```python
from build123d import *

# Parameters (mm, degrees)
CYLINDER001_R     = 5
CYLINDER001_DEPTH = 1.5
CYLINDER002_R     = 2.2
CYLINDER002_DEPTH = 5
CYLINDER_R        = 3
CYLINDER_DEPTH    = 5


with BuildPart() as cylinder001:
    # Cylinder001 → Cylinder001 (new body)
    with BuildSketch(Plane.XY.offset(5)):
        Circle(CYLINDER001_R)
    extrude(amount=CYLINDER001_DEPTH)


with BuildPart() as cylinder002:
    # Cylinder002 → Cylinder002 (new body)
    with BuildSketch(Plane.XY):
        Circle(CYLINDER002_R)
    extrude(amount=CYLINDER002_DEPTH)


with BuildPart() as fusion001:
    # Cylinder → Cylinder (new body)
    with BuildSketch(Plane.XY):
        Circle(CYLINDER_R)
    extrude(amount=CYLINDER_DEPTH)

    # Cut: cut Cylinder002
    add(cylinder002.part, mode=Mode.SUBTRACT)

    # Fusion: union Cylinder001
    add(cylinder001.part)


solid = fusion001.part
```
CAD build for the part. Positions are in the model's coordinates, mm. A direction names the side the tool comes from. Round coordinates to 2 decimals unless told otherwise and drop trailing zeros. Write each loop counter-clockwise with the first axis right and the second up, starting at its lowest first coordinate (ties: lowest second). Pieces come first, ordered by that corner, then holes. Notation, with made-up numbers: (78.25, 45) -> (124.25, 45) arc R18 cw to (124.25, 55) -> close; hole circle Ø7 at (60.25, -18.5). An arc over 180 degrees is marked (long way). Answer in a Markdown table with one row per item. Add a question column.
Item 1: Saw through at D-D, the plane y = 1.25. Write the cut outline in (x, z), then the cut area to 3 significant figures.
Item 2: Saw through at A-A, the plane x = 0. Write the cut outline in (y, z).
Item 3: Drill centre lines: line 1 (Y direction, x = 0, z = 3.8); line 2 (Z direction, x = -1.25, y = -3.25); line 3 (Y direction, x = -1.75, z = 4). Where is each one in solid material? Low to high. Write a range as from..to.
Item 4: Saw through at C-C, the plane z = 3.5. Write the cut outline in (x, y), then the cut area to 3 significant figures.
Item 5: Drop flat-ended pins along their axis: pin 1 Ø1.5 at (y, z) = (-1, 5.5) entering from +X; pin 2 Ø3.5 at (x, y) = (0, 0) entering from -Z; pin 3 Ø1 at (y, z) = (0, 4) entering from +X. Give the stop position or say it passes through.
Item 6: Saw through at B-B, the plane y = -2.75. Write the cut outline in (x, z).
Item 7: Mould opens along X. For faces 3 (the face through (-0.1, -3.3, 5)), 4 (the face through (-3, 0, 2)), 5 (the face through (2.1, 0.66, 2.46)) say: pulls with the +X half, pulls with the -X half, needs draft (parallel to the pull), parting line crosses it, or undercut.
Item 8: Which spindle directions (+Z, -Z, +X, -X, +Y, -Y) get a long thin tool onto all of the face, cutting with end or side? Do faces 1 (the face through (0, 0, 5)), 2 (the face through (0, 0, 6.5)). Say none if no direction does.
Findings below:
| question | item | result |
|---|---|---|
| 1 | outline | (-4.84, 5) -> (-2.73, 5) -> (-2.73, 0) -> (-1.81, 0) -> (-1.81, 5) -> (1.81, 5) -> (1.81, 0) -> (2.73, 0) -> (2.73, 5) -> (4.84, 5) -> (4.84, 6.5) -> (-4.84, 6.5) -> close |
| 1 | area | 23.7 mm^2 |
| 2 | outline | (-5, 5) -> (-3, 5) -> (-3, 0) -> (-2.2, 0) -> (-2.2, 5) -> (2.2, 5) -> (2.2, 0) -> (3, 0) -> (3, 5) -> (5, 5) -> (5, 6.5) -> (-5, 6.5) -> close |
| 3 | line 1 | y = -3..-2.2, 2.2..3 |
| 3 | line 2 | z = 5..6.5 |
| 3 | line 3 | y = -2.44..-1.33, 1.33..2.44 |
| 4 | outline | circle Ø6 at (0, 0); hole circle Ø4.4 at (0, 0) |
| 4 | area | 13.1 mm^2 |
| 5 | pin 1 | stops at x = 4.99 |
| 5 | pin 2 | stops at z = 5 |
| 5 | pin 3 | stops at x = 3 |
| 6 | outline | (-4.18, 5) -> (-1.2, 5) -> (-1.2, 0) -> (1.2, 0) -> (1.2, 5) -> (4.18, 5) -> (4.18, 6.5) -> (-4.18, 6.5) -> close |
| 7 | face 3 | needs draft |
| 7 | face 4 | parting line crosses it |
| 7 | face 5 | undercut |
| 8 | face 1 | -Z |
| 8 | face 2 | +Z, +X, -X, +Y, -Y |
